```python
from build123d import *

# Parameters (mm, degrees)
F0_R     = 76.2
F1_DEPTH = 152.4
F2_R     = 76.2
F3_DEPTH = 76.2
F5_DEPTH = 76.2
F7_DEPTH = 76.2
F9_DEPTH = 76.2


with BuildPart() as f1:
    # F0 (on Top) → F1 (new body)
    with BuildSketch(Plane.XY):
        with BuildLine():
            ThreePointArc((-102.8660584411, 112.447027621), (-77.9844038606, 130.9358344935), (-49.8762557284, 144.0073578485))
            Line((-49.8762557284, 144.0073578485), (-51.4895025042, 146.7159996073))
            Line((-51.4895025042, 146.7159996073), (-103.4791050779, 234.0065559363))
            Line((-103.4791050779, 234.0065559363), (-156.4689077906, 202.4462257088))
            Line((-156.4689077906, 202.4462257088), (-104.4793052169, 115.1556693797))
            Line((-104.4793052169, 115.1556693797), (-102.8660584411, 112.447027621))
        make_face()
        with BuildLine():
            ThreePointArc((149.6603896108, -28.7667826068), (151.7135514328, -14.4484709107), (152.4, 0))
            ThreePointArc((152.4, 0), (151.5011019534, 16.5280400202), (148.8150117204, 32.8611059867))
            ThreePointArc((148.8150117204, 32.8611059867), (74.4015570068, 133.004392089), (-49.8762557284, 144.0073578485))
            ThreePointArc((-49.8762557284, 144.0073578485), (-77.9844038606, 130.9358344935), (-102.8660584411, 112.447027621))
            ThreePointArc((-102.8660584411, 112.447027621), (-152.3859608674, -2.0685575955), (-99.7759023645, -115.1977834307))
            ThreePointArc((-99.7759023645, -115.1977834307), (-74.4015570068, -133.004392089), (-45.9489532793, -145.3081336077))
            ThreePointArc((-45.9489532793, -145.3081336077), (78.0031225642, -130.9246839608), (149.6603896108, -28.7667826068))
        make_face()
        Circle(F0_R, mode=Mode.SUBTRACT)
        with BuildLine():
            Line((-47.4880824642, -148.0595671774), (-45.9489532793, -145.3081336077))
            ThreePointArc((-45.9489532793, -145.3081336077), (-74.4015570068, -133.004392089), (-99.7759023645, -115.1977834307))
            Line((-99.7759023645, -115.1977834307), (-101.3150315494, -117.9492170005))
            Line((-101.3150315494, -117.9492170005), (-150.916069554, -206.6188117265))
            Line((-150.916069554, -206.6188117265), (-97.0891204688, -236.7291619034))
            Line((-97.0891204688, -236.7291619034), (-47.4880824642, -148.0595671774))
        make_face()
        with BuildLine():
            ThreePointArc((148.8150117204, 32.8611059867), (151.5011019534, 16.5280400202), (152.4, 0))
            ThreePointArc((152.4, 0), (151.7135514328, -14.4484709107), (149.6603896108, -28.7667826068))
            Line((149.6603896108, -28.7667826068), (152.8045340537, -28.7667826068))
            Line((152.8045340537, -28.7667826068), (254.3951746319, -27.3877442098))
            Line((254.3951746319, -27.3877442098), (253.5580282594, 34.2829361947))
            Line((253.5580282594, 34.2829361947), (151.9673876811, 32.9038977977))
            Line((151.9673876811, 32.9038977977), (148.8150117204, 32.8611059867))
        make_face()
    extrude(amount=F1_DEPTH)

    # F2 (on face) → F3 (cut)
    with BuildSketch(Plane(origin=(0, 0, 0), x_dir=(1, 0, 0), z_dir=(0, 0, -1))):
        with BuildLine():
            ThreePointArc((148.8150117204, -32.8611059867), (151.5011019534, -16.5280400202), (152.4, 0))
            ThreePointArc((152.4, 0), (151.7135514328, 14.4484709107), (149.6603896108, 28.7667826068))
            ThreePointArc((149.6603896108, 28.7667826068), (78.0031225642, 130.9246839608), (-45.9489532793, 145.3081336077))
            ThreePointArc((-45.9489532793, 145.3081336077), (-74.4015570068, 133.004392089), (-99.7759023645, 115.1977834307))
            ThreePointArc((-99.7759023645, 115.1977834307), (-152.3859608674, 2.0685575955), (-102.8660584411, -112.447027621))
            ThreePointArc((-102.8660584411, -112.447027621), (-77.9844038606, -130.9358344935), (-49.8762557284, -144.0073578485))
            ThreePointArc((-49.8762557284, -144.0073578485), (74.4015570068, -133.004392089), (148.8150117204, -32.8611059867))
        make_face()
        Circle(F2_R, mode=Mode.SUBTRACT)
        Circle(F2_R)
    extrude(amount=-F3_DEPTH, mode=Mode.SUBTRACT)

    # F4 (on face) → F5 (cut)
    with BuildSketch(Plane(origin=(-0.4185731863, 30.8353402022, 0), x_dir=(-0.9999078797, -0.0135732126, 0), z_dir=(-0.0135732126, 0.9999078797, 0))):
        Polygon((-254, 38.1), (-149.2473336147, 152.4), (-254, 152.4), align=None)
        Polygon((-149.2473336147, 0), (-149.2473336147, 76.2), (-241.3, 0), align=None)
    extrude(amount=-F5_DEPTH, mode=Mode.SUBTRACT)

    # F6 (on face) → F7 (cut)
    with BuildSketch(Plane(origin=(-26.4949013563, -15.7801651138, 0), x_dir=(0.5117086867, -0.859159019, 0), z_dir=(-0.859159019, -0.5117086867, 0))):
        Polygon((-254, 38.1), (-149.2473336147, 152.4), (-254, 152.4), align=None)
        Polygon((-149.2473336147, 0), (-149.2473336147, 76.2), (-241.3, 0), align=None)
    extrude(amount=-F7_DEPTH, mode=Mode.SUBTRACT)

    # F8 (on face) → F9 (cut)
    with BuildSketch(Plane(origin=(26.9134745426, -15.0551750885, 0), x_dir=(0.488199193, 0.8727322316, 0), z_dir=(0.8727322316, -0.488199193, 0))):
        Polygon((-254, 38.1), (-149.2473336147, 152.4), (-254, 152.4), align=None)
        Polygon((-149.2473336147, 0), (-149.2473336147, 76.2), (-241.3, 0), align=None)
    extrude(amount=-F9_DEPTH, mode=Mode.SUBTRACT)


solid = f1.part
```
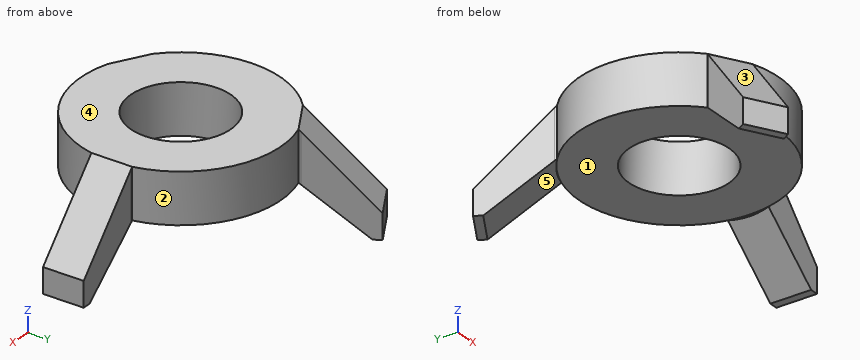
Build history of the part. All positions in model axes, mm. Face numbers are marked on the shaded views. A direction names the side the tool comes from. Give positions to 0.01 mm unless a question says otherwise; leave off trailing zeros. Loops run counter-clockwise (first coordinate to the right, second up) from the corner with the lowest first, then second, coordinate; pieces in that order, holes last.
Item 1: Slice it at C-C, the plane x = -114.5. List the corners of the cut face in (y, z).
Answers follow:
outline: (-226.99, 0) - (-212.44, 0) - (-141.52, 51.23) - (-141.52, 119.49) - (-226.99, 38.1) - close; (-100.58, 76.2) - (100.58, 76.2) - (100.58, 152.4) - (-100.58, 152.4) - close; (131.98, 57.38) - (212.66, 0) - (227.44, 0) - (227.44, 38.1) - (131.98, 127.59) - close
Item 2: Slice it at D-D, the plane z = 101. List the corners of the cut face in (x, y), and give its area (3 significant figures).
Answers follow:
outline: (-126.97, 152.92) - (-102.87, 112.45) arc R152.4 ccw to (-99.78, -115.2) - (-122.77, -156.31) - (-68.95, -186.42) - (-45.95, -145.31) arc R152.4 ccw to (149.66, -28.77) - (152.8, -28.77) - (196.75, -28.17) - (195.92, 33.5) - (148.82, 32.86) arc R152.4 ccw to (-49.88, 144.01) - (-73.98, 184.48) - close; hole circle Ø152.4 at (0, 0)
area: 63,100 mm2
Item 3: Flat gauge pins, fed straight in: pin 1 (5 mm diameter, centred on x = 85.5, z = 111, fed in from -Y); pin 2 (1.5 mm diameter, centred on x = 173.5, z = 95, fed in from -Y); pin 3 (6 mm diameter, centred on x = 157, z = 79, fed in from +Y). Where does each tip first touch, or does it go through?
Answers follow:
pin 1: stops at y = -127.82
pin 2: stops at y = -28.5
pin 3: stops at y = 33.01
Item 4: Which spindle directions (+Z, -Z, +X, -X, +Y, -Y) get a long thin tool onto all of the face, cutting with end or side? Do the marked faces 4 and 5. Say none if no direction does.
Answers follow:
face 4: +Z, +X, -X, +Y, -Y
face 5: -Z, +X
Item 5: Slice it at B-B, the plane z = 24. List the corners of the cut face in (x, y).
Answers follow:
outline: (-156.47, 202.45) - (-135.13, 166.63) - (-82.14, 198.19) - (-103.48, 234.01) - close; (-150.92, -206.62) - (-97.09, -236.73) - (-76.73, -200.34) - (-130.56, -170.23) - close; (211.87, 33.72) - (212.71, -27.95) - (254.4, -27.39) - (253.56, 34.28) - close
Item 6: Slice it at A-A, the plane x = 0. List the corners of the cut face in (y, z), and give its area (3 significant figures).
Answers follow:
outline: (-152.4, 76.2) - (-76.2, 76.2) - (-76.2, 152.4) - (-152.4, 152.4) - close; (76.2, 76.2) - (152.4, 76.2) - (152.4, 152.4) - (76.2, 152.4) - close
area: 11,600 mm2
Item 7: Drill centre lines: line 1 (Y direction, x = 0, z = 131); line 2 (Z direction, x = 119, y = 76); line 3 (X direction, y = 0, z = 101). Where is each one in solid material? Low to high.
Answers follow:
line 1: y = -152.4 to -76.2, 76.2 to 152.4
line 2: z = 76.2 to 152.4
line 3: x = -152.4 to -76.2, 76.2 to 196.37
Item 8: Pull direction Y, two halves, no side cores. Call the marked faces 1, 2 and 3: released by +Y, released by -Y, zero draft, split by the parting line, or undercut.
Answers follow:
face 1: undercut
face 2: released by +Y
face 3: released by -Y
